Model file for the job. Use its own axes, mm. Coordinates: 2 decimals unless noted, no trailing zeros. Write each loop counter-clockwise with the first axis right and the second up, starting at its lowest first coordinate (ties: lowest second). Pieces come first, ordered by that corner, then holes. Notation, with made-up numbers: M 48,77 L 54,77 A19 ccw 54,98 Z; hole C 5,80 d1. An arc over 180 degrees is marked long. Use CSV: the item, a comma, the result in double quotes. Start each with the question number.
Autodesk Fusion 360 part; units mm, degrees
sketch "スケッチ1" plane through (0, 0, 0) normal (0, 0, 1) x (1, 0, 0)
  line L0 (-15.5, 115) -> (-74.5, 115)
  line L1 (-74.5, 115) -> (-74.5, -115)
  line L2 (-74.5, -115) -> (-15.5, -115)
  line L3 (74.5, -75) -> (74.5, 105)
  line L4 (68.0217, 105) -> (-74.5, -115) construction
  line L5 (-74.5, 115) -> (54.38, -83.9422) construction
  line L6 (-15.5, 115) -> (-15.5, 105)
  line L7 (-15.5, 105) -> (74.5, 105)
  line L8 (-74.5, -115) -> (-15.5, -115) construction
  line L9 (74.5, -75) -> (-15.5, -115)
  dimension "d2" = 230
  dimension "d5" = 59
extrude "押し出し1" add sketch "スケッチ1" along normal blind 6
chamfer "面取り1" distance 20 angle 45 2 edges at (-74.5, -115, 3) (-74.5, 115, 3)
sketch "スケッチ2" plane through (0, 0, 6) normal (0, 0, 1) x (-1, 0, 0)
  line L0 (54.5, -115) -> (74.5, -95)
  line L1 (74.5, -95) -> (74.5, 95)
  line L2 (74.5, 95) -> (54.5, 115)
  line L3 (54.5, 115) -> (15.5, 115)
  line L4 (15.5, 115) -> (-74.5, 75)
  line L5 (-74.5, 75) -> (-74.5, -105)
  line L6 (-74.5, -105) -> (15.5, -105)
  line L7 (15.5, -105) -> (15.5, -115)
  line L8 (15.5, -115) -> (54.5, -115)
  line L9 (-74.5, -105) -> (-34.5, -105) construction
  line L10 (-34.5, -105) -> (-34.5, -55) construction
  line L11 (-34.5, -55) -> (-74.5, -55) construction
  line L12 (-74.5, -55) -> (-74.5, -105) construction
  line L13 (-34.5, -55) -> (-34.5, 5) construction
  point P0 (-34.5, -55)
  point P1 (-34.5, 5)
  dimension "d10" = 40
  dimension "d11" = 50
  dimension "d12" = 60
hole "穴1" at (34.5, 55, 6) at (34.5, -5, 6) direction (0, 0, -1) diameter 18 end through all
equation "d5 = 20 mm + 39 mm"
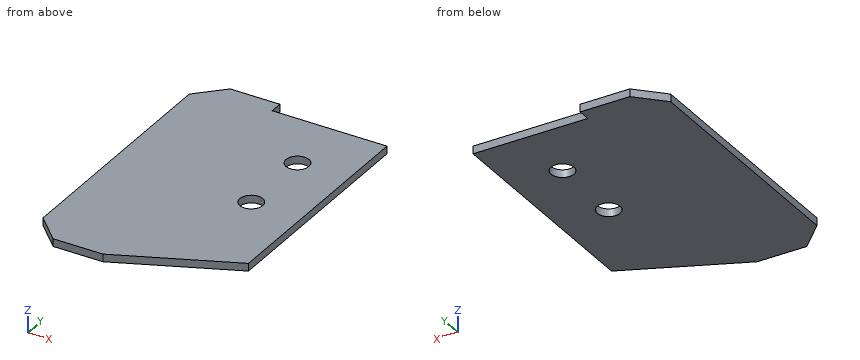
1) Band-saw the part on D-D on x = 51.5. List the corners of the cut face in (y, z).
2) Band-saw the part on B-B on z = 1. List the corners of the cut face in (x, y).
3) Band-saw the part on C-C on x = 34.5. List the corners of the cut face in (y, z).
4) Band-saw the part on A-A on y = 55. List the corners of the cut face in (x, z).
5) Drop flat-ended pins along their axis: P1, Ø1.5, axis at y = -87.5, z = 4, coming from the +X side; P2, Ø1.8, axis at y = 111, z = 3.5, coming from the +X side. Give the stop position or say it passes through.
6) Wall check: L1, parallel to Y at x = 34.5, z = 3.45; L2, parallel to Y at x = 36, z = 3.35; L3, parallel to X at y = 55, z = 4.25. Give the ranges that are in metal, low to high. Write a range as [from, to].
Findings below:
1,outline,"M -85.22,0 L 105,0 L 105,6 L -85.22,6 Z"
2,outline,"M -74.5,-95 L -54.5,-115 L -15.5,-115 L 74.5,-75 L 74.5,105 L -15.5,105 L -15.5,115 L -54.5,115 L -74.5,95 Z; hole C 34.5,-5 d18; hole C 34.5,55 d18"
3,outline,"M -92.78,0 L -14,0 L -14,6 L -92.78,6 Z; M 4,0 L 46,0 L 46,6 L 4,6 Z; M 64,0 L 105,0 L 105,6 L 64,6 Z"
4,outline,"M -74.5,0 L 25.5,0 L 25.5,6 L -74.5,6 Z; M 43.5,0 L 74.5,0 L 74.5,6 L 43.5,6 Z"
5,P1,"stops at x = 48.06"
5,P2,"stops at x = -15.5"
6,L1,"y = [-92.78, -14], [4, 46], [64, 105]"
6,L2,"y = [-92.11, -13.87], [3.87, 46.13], [63.87, 105]"
6,L3,"x = [-74.5, 25.5], [43.5, 74.5]"
